Here's the drawing with two shaded views (mm, measured from the low corner). I have some questions. A direction names the side the tool comes from. Round coordinates to 2 decimals unless told otherwise and drop trailing zeros. Loops run counter-clockwise (first coordinate to the right, second up) from the corner with the lowest first, then second, coordinate; pieces in that order, holes last. Notation, with made-up numbers: (-10, -27.5) - (8, -27.5) arc R17 ccw to (8, 0.5) - close; hole circle Ø1 at (59, 49). An arc over 180 degrees is marked (long way). Use one line per item in the form item = value.
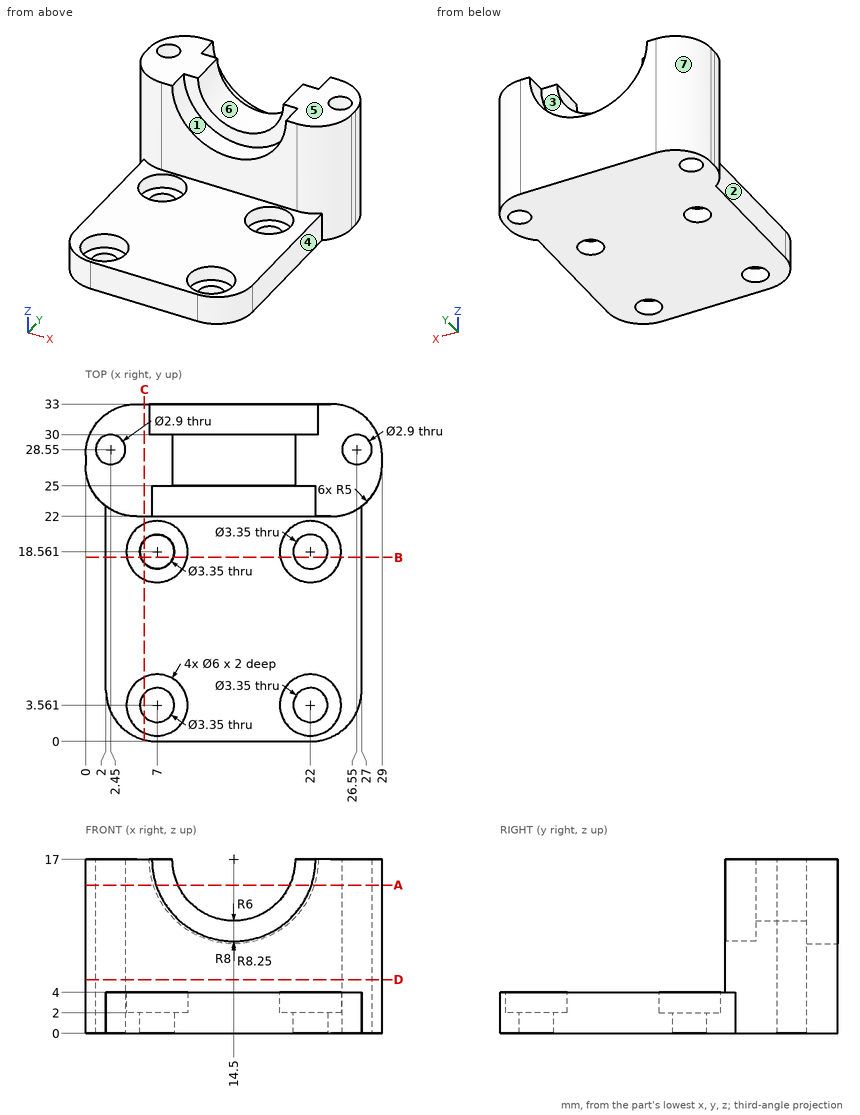
1. For P1, Ø4, axis at x = 22, y = 18.56, coming from the -Z side; P2, Ø5, axis at y = 10.5, z = 8.5, coming from the +X side; P3, Ø9, axis at x = 12, z = 11.5, coming from the -Y side; P4, Ø3, axis at x = 21, y = 4, coming from the +Z side, each with a flat end and sliding along its axis, tell me the tip position at first contact or that it passes through.
Solution:
P1 = 0
P2 = through
P3 = 22
P4 = 2
2. If we section it at D-D, the plane z = 5.25: Write out the boundary of the cut face in (x, y).
Solution:
outline = (0, 27) arc R5 ccw to (5, 22) - (24, 22) arc R5 ccw to (29, 27) - (29, 28) arc R5 ccw to (24, 33) - (5, 33) arc R5 ccw to (0, 28) - close; hole circle Ø2.9 at (2.45, 28.55); hole circle Ø2.9 at (26.55, 28.55)
3. Please list where these lines run through material, in increasing order: line 1 along Y through (x, z) = (7, 0.95) (1 decimal); line 2 along X through (y, z) = (29, 15); line 3 along X through (y, z) = (27, 12.75) (1 decimal).
Solution:
line_1 = 0 to 1.9, 5.2 to 16.9, 20.2 to 33
line_2 = 0.1 to 1.07, 3.83 to 8.84, 20.16 to 25.17, 27.93 to 28.9
line_3 = 0 to 10.3, 18.7 to 29
4. If we section it at A-A, the plane z = 14.5: Count the separate pieces of the cut face and the enclosed holes in it, plus the area to 3 significant figures.
Solution:
separate_pieces = 2
enclosed_holes = 2
area = 137 mm^2
5. If we section it at C-C, the plane x = 5.75: Write out the boundary of the cut face in (y, z) (1 decimal).
Solution:
outline = (0.2, 0) - (2.4, 0) - (2.4, 2) - (0.8, 2) - (0.8, 4) - (0.2, 4) - close; (4.7, 0) - (17.4, 0) - (17.4, 2) - (15.8, 2) - (15.8, 4) - (6.3, 4) - (6.3, 2) - (4.7, 2) - close; (19.7, 0) - (33, 0) - (33, 17) - (22, 17) - (22, 4) - (21.3, 4) - (21.3, 2) - (19.7, 2) - close
6. We'd pull the mould along X, two halves only. Please class the marked faces 5, 6 and 7: +X half, -X half, draft (parallel to the pull), parting line (faces both ways), or undercut.
Solution:
face_5 = draft
face_6 = undercut
face_7 = -X half
7. On a 3-axis mill with a long thin cutter (end or side, diameter ignored), from which of +Z, -Z, +X, -X, +Y, -Y can I reach the whole of each face in a straight line? I mean the marked faces 1, 2, 3 and 4. Say none if no direction works.
Solution:
face_1 = +Z, -Y
face_2 = +Z, -Z, -X, -Y
face_3 = +Z, +Y
face_4 = +Z, -Z, +X, -Y
8. If we section it at B-B, the plane y = 18: Write out the boundary of the cut face in (x, z).
Solution:
outline = (2, 0) - (5.42, 0) - (5.42, 2) - (4.05, 2) - (4.05, 4) - (2, 4) - close; (8.58, 0) - (20.42, 0) - (20.42, 2) - (19.05, 2) - (19.05, 4) - (9.95, 4) - (9.95, 2) - (8.58, 2) - close; (23.58, 0) - (27, 0) - (27, 4) - (24.95, 4) - (24.95, 2) - (23.58, 2) - close
